Check sheet for the drawn part. Datum: minimum x, y, z corner. Units: mm. Coordinates: 2 decimals unless noted, no trailing zeros. Write each loop counter-clockwise with the first axis right and the second up, starting at its lowest first coordinate (ties: lowest second). Pieces come first, ordered by that corner, then holes. Notation, with made-up numbers: (-15, -31) -> (42, -31) arc R9 ccw to (42, -15) -> close; hole circle Ø8 at (-19, -25). An arc over 180 degrees is marked (long way). Answer in a Markdown table with one row per item.
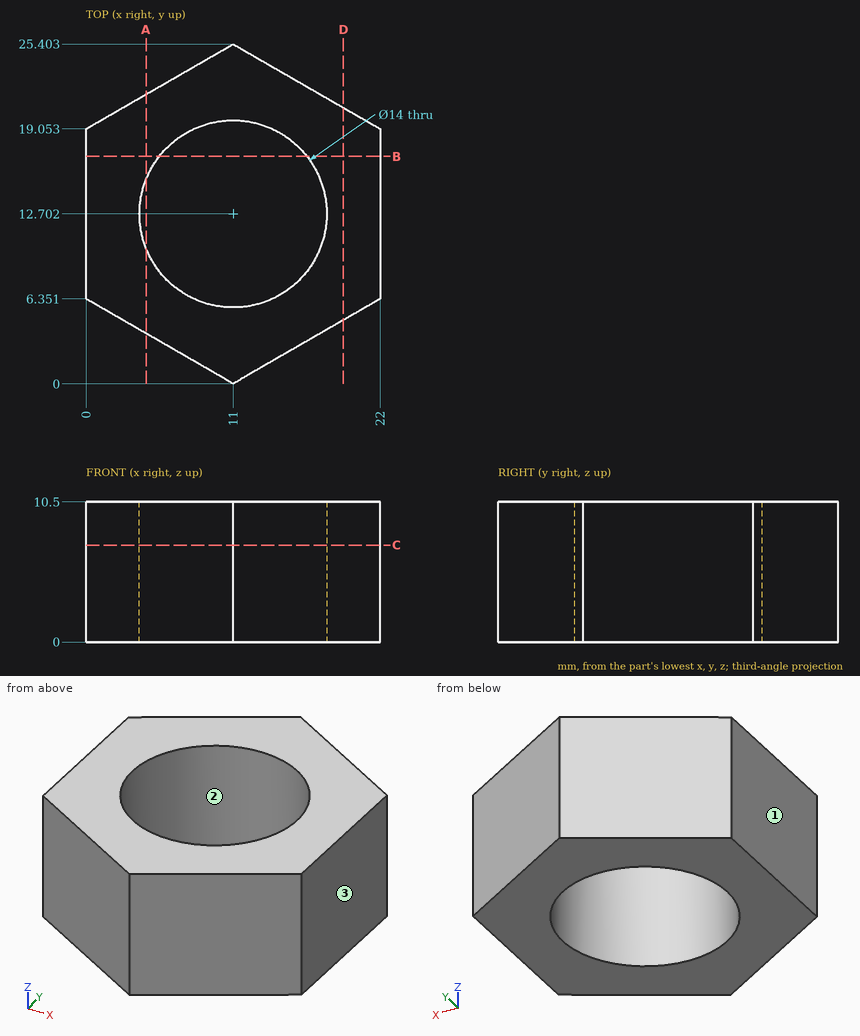
1. Sectioned sample at A-A, the plane x = 4.5. Record the cut outline in (y, z), and give its area (3 significant figures).
Findings below:
| item | result |
|---|---|
| outline | (3.75, 0) -> (10.1, 0) -> (10.1, 10.5) -> (3.75, 10.5) -> close; (15.3, 0) -> (21.65, 0) -> (21.65, 10.5) -> (15.3, 10.5) -> close |
| area | 133 mm² |
2. Sectioned sample at B-B, the plane y = 17. Record the cut outline in (x, z) (1 decimal).
Findings below:
| item | result |
|---|---|
| outline | (0, 0) -> (5.5, 0) -> (5.5, 10.5) -> (0, 10.5) -> close; (16.5, 0) -> (22, 0) -> (22, 10.5) -> (16.5, 10.5) -> close |
3. Go/stop test with flat-tipped pins: pin 1 (8.5 mm diameter, centred on x = 11, y = 12.7, fed in from +Z); pin 2 (5 mm diameter, centred on x = 4.5, z = 8.5, fed in from +Y) (1 decimal); pin 3 (3 mm diameter, centred on y = 4, z = 4, fed in from +X) (1 decimal). Record where each tip stops, or that it passes through.
Findings below:
| item | result |
|---|---|
| pin 1 | passes through |
| pin 2 | stops at y = 23.1 |
| pin 3 | stops at x = 20.5 |
4. Material ranges on probe 1 along X at (y, z) = (7.5, 2) (1 decimal); probe 2 along X at (y, z) = (11.5, 2.75) (1 decimal); probe 3 along Y at (x, z) = (12, 9.25) (1 decimal), recorded low to high. Write a range as from..to.
Findings below:
| item | result |
|---|---|
| probe 1 | x = 0..6.3, 15.7..22 |
| probe 2 | x = 0..4.1, 17.9..22 |
| probe 3 | y = 0.6..5.8, 19.6..24.8 |
5. Sectioned sample at D-D, the plane x = 19.25. Record the cut outline in (y, z), and give its area (3 significant figures).
Findings below:
| item | result |
|---|---|
| outline | (4.76, 0) -> (20.64, 0) -> (20.64, 10.5) -> (4.76, 10.5) -> close |
| area | 167 mm² |
6. Sectioned sample at C-C, the plane z = 7.25. Record the cut outline in (x, y), and give its area (3 significant figures).
Findings below:
| item | result |
|---|---|
| outline | (0, 6.35) -> (11, 0) -> (22, 6.35) -> (22, 19.05) -> (11, 25.4) -> (0, 19.05) -> close; hole circle Ø14 at (11, 12.7) |
| area | 265 mm² |
7. Release check for a two-part mould opening along X. For the marked faces 1, 2 and 3 record: released by +X, released by -X, zero draft, split by the parting line, or undercut.
Findings below:
| item | result |
|---|---|
| face 1 | released by -X |
| face 2 | undercut |
| face 3 | released by +X |
